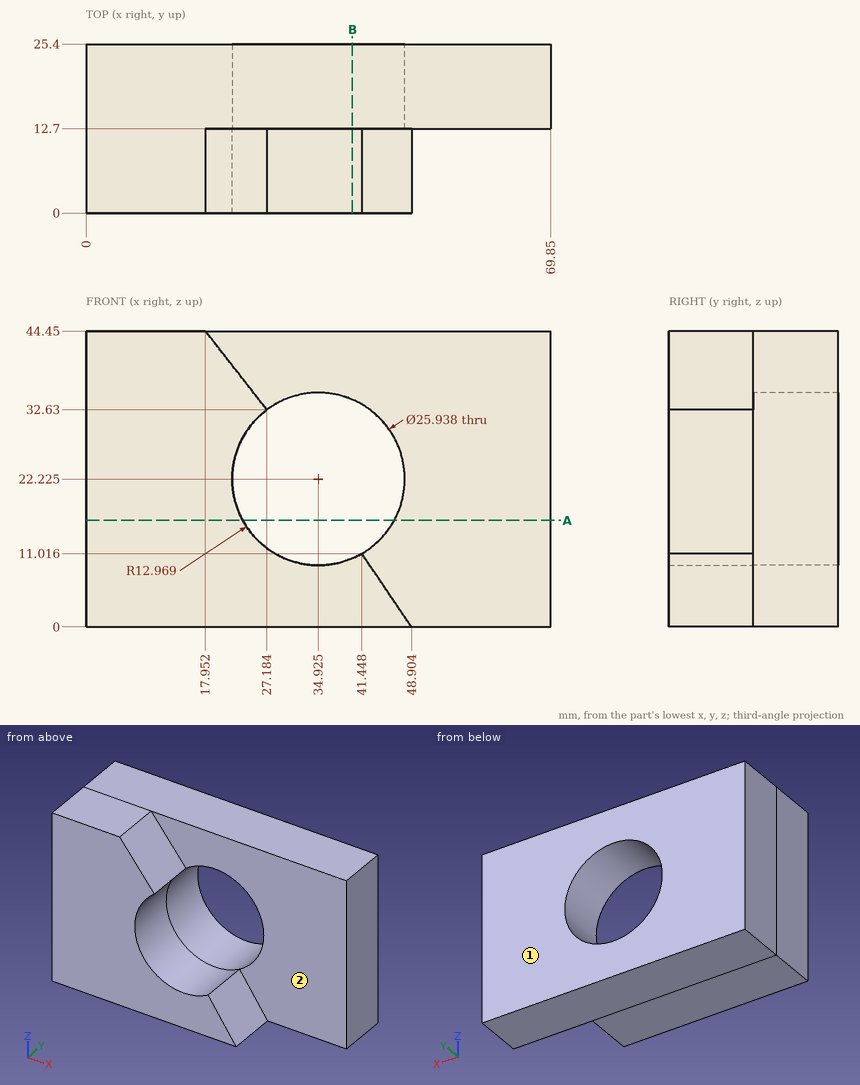
Job drawing, mm, ordinate dimensions from the low corner. One solid piece. A direction names the side the tool comes from. Round coordinates to 2 decimals unless told otherwise and drop trailing zeros. Order: outer loops, then holes, each group sorted by start corner. A loop starts at its lowest first (then second) coordinate and runs counter-clockwise, first axis right, second up. Notation, with made-up numbers: (22.25, 39) -> (74.25, 39) arc R20 cw to (74.25, 49) -> close; hole circle Ø9 at (79.25, 51.25). An arc over 180 degrees is marked (long way). Write item = value, one per line.
(1) Cut at A-A (z = 16). Write the cut outline in (x, y).
Answers follow:
outline = (0, 0) -> (23.55, 0) -> (23.55, 25.4) -> (0, 25.4) -> close; (46.3, 12.7) -> (69.85, 12.7) -> (69.85, 25.4) -> (46.3, 25.4) -> close
(2) Flat gauge pins, fed straight in: P1, Ø6, axis at y = 6, z = 34.5, coming from the +X side; P2, Ø6, axis at x = 60, z = 8, coming from the -Y side; P3, Ø6, axis at y = 3, z = 17, coming from the +X side. Where does each tip first touch, or does it go through?
Answers follow:
P1 = 27.18
P2 = 12.7
P3 = 24.9
(3) Drill centre lines: L1, parallel to Y at x = 58.5, z = 10.5; L2, parallel to X at y = 13.25, z = 14; L3, parallel to X at y = 16.5, z = 26. Where is each one in solid material? Low to high.
Answers follow:
L1 = 12.7 to 25.4
L2 = 0 to 24.9, 44.95 to 69.85
L3 = 0 to 22.52, 47.33 to 69.85
(4) 3-axis set-ups, long thin cutter, end or side, ignore diameter. For the marked faces 1 and 2: which of +Z, -Z, +X, -X, +Y, -Y reach the whole face in a straight line?
Answers follow:
face_1 = +Z, -Z, +X, -X, +Y
face_2 = +Z, +X, -Y
(5) Cut at B-B (x = 40). Write the cut outline in (y, z).
Answers follow:
outline = (0, 0) -> (25.4, 0) -> (25.4, 10.29) -> (0, 10.29) -> close; (12.7, 34.16) -> (25.4, 34.16) -> (25.4, 44.45) -> (12.7, 44.45) -> close
